For this review, take the finished solid that the model builds, in its own axes (mm). Coordinates: 2 decimals unless noted, no trailing zeros. Write each loop counter-clockwise with the first axis right and the second up, starting at its lowest first coordinate (ties: lowest second). Pieces come first, ordered by that corner, then holes. Notation, with made-up numbers: (31.25, -27.5) -> (82.25, -27.5) arc R11 cw to (82.25, -20.5) -> close; hole circle Ø9 at (53, 83.5). An arc over 180 degrees is marked (long way). Put each result on its own line as item: value. Start each with the question number.
Item 1: Consider section D-D on x = 33.5. Give the boundary of the cut face in (y, z), and give its area (3 significant figures).
Item 2: To check wall thickness, follow L1, parallel to Y at x = 14, z = 0.75; L2, parallel to Y at x = 14.5, z = 4.65; L3, parallel to Y at x = 28, z = 3.9. State the ranges of each line that lie inside material, in increasing order.
Item 3: Insertion check: P1, Ø2, axis at x = 5.5, y = 6, coming from the -Z side; P2, Ø1, axis at x = 15.5, z = 2, coming from the +Y side. Each pin has a flat end and moves straight along its axis. Give the tip position at first contact, or say it passes through.
Item 4: Consider section C-C on z = 2.3. Give the boundary of the cut face in (x, y), and give its area (3 significant figures).
Item 5: Consider section B-B on y = 7.5. Give the boundary of the cut face in (x, z), and give its area (3 significant figures).
Item 6: Consider section A-A on x = 13.5. Give the boundary of the cut face in (y, z), and give its area (3 significant figures).
Item 7: The part is to be moulded in two halves that separate along Y. For faces 1 (the cylindrical face through (1.31, 7.22, 2.46)), 2 (the cylindrical face through (17, 4.65, 2.46)), 3 (the flat face through (15.3, 1.7, 0)), 4 (the flat face through (21.587, 4.934, 2.465)), say which applies: +Y half, -Y half, draft (parallel to the pull), parting line (faces both ways), or undercut.
```python
from build123d import *

# Parameters (mm, degrees)
SKETCH_8_R      = 2.1
EXTRUDE_6_DEPTH = 5


with BuildPart() as part:
    # 草图8 → 凸台-拉伸6 (new body)
    with BuildSketch(Plane.XY):
        Polygon((0, 0), (40, 0), (2.651084003, 10.00761403), (0, 8.558252816), align=None)
        with Locations((3.406885567, 7.12453076)):
            Circle(SKETCH_8_R, mode=Mode.SUBTRACT)
        with Locations((14.997995315, 4.018701596)):
            Circle(SKETCH_8_R, mode=Mode.SUBTRACT)
    extrude(amount=EXTRUDE_6_DEPTH)


solid = part.part
```
Return value:
1. outline: (0, 0) -> (1.74, 0) -> (1.74, 5) -> (0, 5) -> close
1. area: 8.71 mm^2
2. L1: 0 to 2.17, 5.87 to 6.97
2. L2: 0 to 1.98, 6.06 to 6.83
2. L3: 0 to 3.22
3. P1: z = 0
3. P2: y = 6.7
4. outline: (0, 0) -> (40, 0) -> (2.65, 10.01) -> (0, 8.56) -> close; hole circle Ø4.2 at (3.41, 7.12); hole circle Ø4.2 at (15, 4.02)
4. area: 184 mm^2
5. outline: (0, 0) -> (1.34, 0) -> (1.34, 5) -> (0, 5) -> close; (5.47, 0) -> (12.01, 0) -> (12.01, 5) -> (5.47, 5) -> close
5. area: 39.4 mm^2
6. outline: (0, 0) -> (2.55, 0) -> (2.55, 5) -> (0, 5) -> close; (5.49, 0) -> (7.1, 0) -> (7.1, 5) -> (5.49, 5) -> close
6. area: 20.8 mm^2
7. face 1: undercut
7. face 2: undercut
7. face 3: draft
7. face 4: +Y half
